Job drawing, mm, ordinate dimensions from the low corner. One solid piece. A direction names the side the tool comes from. Give positions to 0.01 mm unless a question says otherwise; leave off trailing zeros. Write each loop counter-clockwise with the first axis right and the second up, starting at its lowest first coordinate (ties: lowest second). Pieces come first, ordered by that corner, then holes. Notation, with made-up numbers: (50, -38.5) - (93, -38.5) arc R23 cw to (93, -10.5) - close; hole circle Ø9 at (19.25, 66). An arc over 180 degrees is marked (long way). Answer as a JSON object with one key per item and string values.
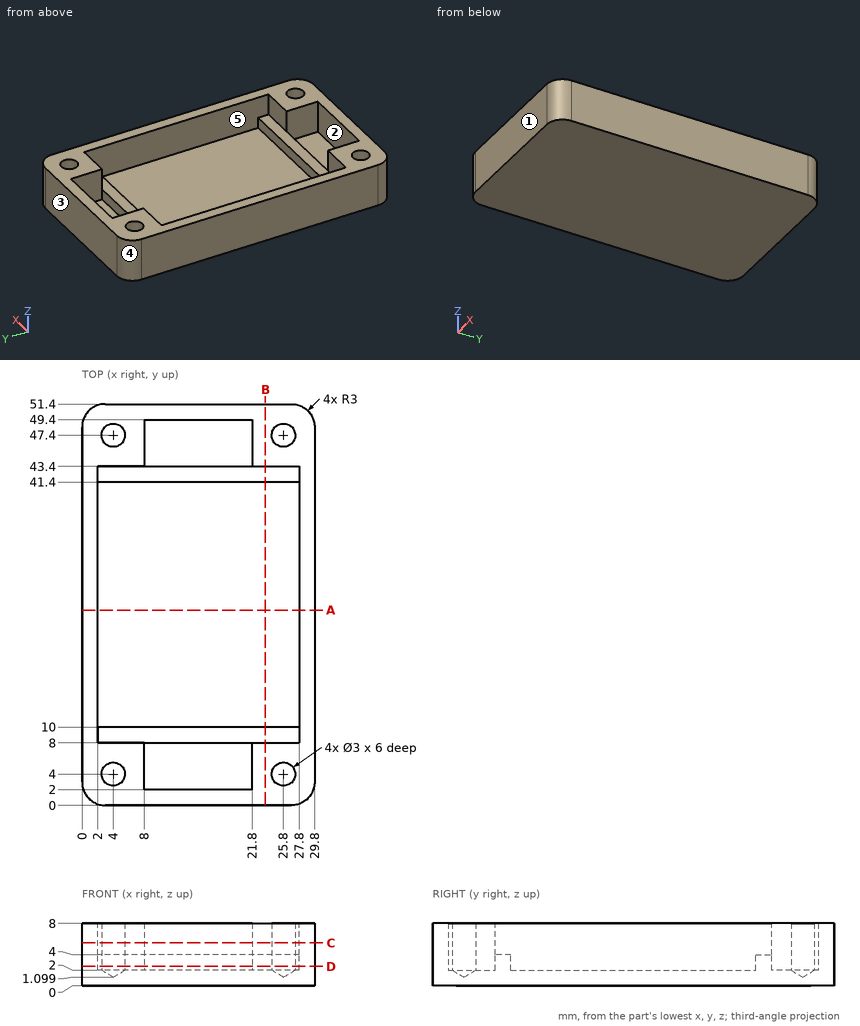
Item 1: Cut at D-D (z = 2.5). Give the cut face in (x, y), and give its area (3 significant figures).
Entries:
{"outline": "(0, 3) arc R3 ccw to (3, 0) - (26.8, 0) arc R3 ccw to (29.8, 3) - (29.8, 48.4) arc R3 ccw to (26.8, 51.4) - (3, 51.4) arc R3 ccw to (0, 48.4) - close; hole (2, 10) - (27.8, 10) - (27.8, 41.4) - (2, 41.4) - close; hole circle Ø3 at (4, 4); hole circle Ø3 at (4, 47.4); hole (8, 2) - (21.8, 2) - (21.8, 8) - (8, 8) - close; hole (8, 43.4) - (21.8, 43.4) - (21.8, 49.4) - (8, 49.4) - close; hole circle Ø3 at (25.8, 4); hole circle Ø3 at (25.8, 47.4)", "area": "520 mm2"}
Item 2: Cut at A-A (y = 25). Give the cut face in (x, z).
Entries:
{"outline": "(0, 0) - (29.8, 0) - (29.8, 8) - (27.8, 8) - (27.8, 2) - (2, 2) - (2, 8) - (0, 8) - close"}
Item 3: Which spindle directions (+Z, -Z, +X, -X, +Y, -Y) get a long thin tool onto all of the face, cutting with end or side? Do the marked faces 4 and 5. Say none if no direction does.
Entries:
{"face 4": "+Z, -Z, -X, +Y", "face 5": "+Z"}
Item 4: Cut at C-C (z = 5.5). Give the cut face in (x, y).
Entries:
{"outline": "(0, 3) arc R3 ccw to (3, 0) - (26.8, 0) arc R3 ccw to (29.8, 3) - (29.8, 48.4) arc R3 ccw to (26.8, 51.4) - (3, 51.4) arc R3 ccw to (0, 48.4) - close; hole (2, 8) - (8, 8) - (8, 2) - (21.8, 2) - (21.8, 8) - (27.8, 8) - (27.8, 43.4) - (21.8, 43.4) - (21.8, 49.4) - (8, 49.4) - (8, 43.4) - (2, 43.4) - close; hole circle Ø3 at (4, 4); hole circle Ø3 at (4, 47.4); hole circle Ø3 at (25.8, 4); hole circle Ø3 at (25.8, 47.4)"}
Item 5: Mould opens along Y. For the marked faces 1, 2 and 3 say: +Y half, -Y half, draft (parallel to the pull), parting line (faces both ways), or undercut.
Entries:
{"face 1": "-Y half", "face 2": "undercut", "face 3": "+Y half"}
Item 6: Probe line 1 (X direction, y = 47.4, z = 5.75); line 2 (Y direction, x = 25.8, z = 4.05); line 3 (X direction, y = 22, z = 2.5). List the from-to ranges inside material, lowest first. Write a range as from..to.
Entries:
{"line 1": "0..2.5, 5.5..8, 21.8..24.3, 27.3..29.8", "line 2": "0..2.5, 5.5..8, 43.4..45.9, 48.9..51.4", "line 3": "0..2, 27.8..29.8"}
Item 7: Flat gauge pin, fed straight in: P1, Ø5, axis at x = 12.5, y = 22, coming from the +Z side. Where does the tip first touch, or does it go through?
Entries:
{"P1": "z = 2"}
Item 8: Cut at B-B (x = 23.5). Give the cut face in (y, z).
Entries:
{"outline": "(0, 0) - (51.4, 0) - (51.4, 8) - (43.4, 8) - (43.4, 4) - (41.4, 4) - (41.4, 2) - (10, 2) - (10, 4) - (8, 4) - (8, 8) - (0, 8) - close"}
